Here's how the part is built. I have some questions about the finished solid (model axes, mm). Coordinates: 2 decimals unless noted, no trailing zeros.
from build123d import *

# Parameters (mm, degrees)
F0_W     = 115
F0_H     = 85
F0_W_2   = 3.3230667468
F0_H_2   = 2.7188727399
F0_W_3   = 12.42488157
F0_H_3   = 2.8554350138
F0_W_4   = 2.7188727399
F0_H_4   = 3.3230667468
F0_W_5   = 2.8554350138
F0_H_5   = 12.42488157
F1_DEPTH = 3
F2_R     = 2.6556349186
F3_D     = 3.3
F3_DEPTH = 13.5
F3_TIP   = 0.9914200214
F4_D     = 3.3


with BuildPart() as f1:
    # F0 (on Top) → F1 (new body)
    with BuildSketch(Plane.XY):
        Rectangle(F0_W, F0_H)
        with Locations((-31.5384735586, -39.6359708975)):
            Rectangle(F0_W_2, F0_H_2, mode=Mode.SUBTRACT)
        with Locations((-23.0330330087, -39.6208088496)):
            Rectangle(F0_W_2, F0_H_2, mode=Mode.SUBTRACT)
        with Locations((0.012440607, -39.7679619491)):
            Rectangle(F0_W_3, F0_H_3, mode=Mode.SUBTRACT)
        with Locations((23.7232622458, -35.9257351956)):
            Rectangle(F0_W_2, F0_H_2, mode=Mode.SUBTRACT)
        with Locations((32.2287027957, -35.9105731477)):
            Rectangle(F0_W_2, F0_H_2, mode=Mode.SUBTRACT)
        with Locations((0.0594367157, -4.1384646902)):
            Rectangle(F0_W_4, F0_H_4, mode=Mode.SUBTRACT)
        with Locations((54.6148940921, -0.0461908057)):
            Rectangle(F0_W_5, F0_H_5, mode=Mode.SUBTRACT)
        with Locations((-54.6360462904, 0)):
            Rectangle(F0_W_5, F0_H_5, mode=Mode.SUBTRACT)
        with Locations((-31.1669755029, 39.4913438358)):
            Rectangle(F0_W_2, F0_H_2, mode=Mode.SUBTRACT)
        with Locations((-22.6615349529, 39.5065058838)):
            Rectangle(F0_W_2, F0_H_2, mode=Mode.SUBTRACT)
        with Locations((0.0442746677, 4.3669758597)):
            Rectangle(F0_W_4, F0_H_4, mode=Mode.SUBTRACT)
        with Locations((0.1124413684, 39.7277288139)):
            Rectangle(F0_W_3, F0_H_3, mode=Mode.SUBTRACT)
        with Locations((23.6730267061, 36.7241497734)):
            Rectangle(F0_W_2, F0_H_2, mode=Mode.SUBTRACT)
        with Locations((32.178467256, 36.7393118213)):
            Rectangle(F0_W_2, F0_H_2, mode=Mode.SUBTRACT)
    extrude(amount=-F1_DEPTH)

    # F2
    f2_edges = [f1.edges().sort_by_distance(p)[0] for p in [
        (57.5, -42.5, -1.5),
        (57.5, 42.5, -1.5),
        (-57.5, -42.5, -1.5),
        (-57.5, 42.5, -1.5),
    ]]
    fillet(f2_edges, radius=F2_R)

    # F3
    with Locations(Plane.XY):
        with Locations((-53.4860491753, -38.9412779514), (-53.4860491753, 39.0123836696), (53.5768903792, -38.9412779514), (53.5768903792, 39.0123836696)):
            Hole(F3_D / 2, depth=F3_DEPTH)
            with Locations((0, 0, -(F3_DEPTH + F3_TIP / 2))):  # 118° drill point
                Cone(0, F3_D / 2, F3_TIP, mode=Mode.SUBTRACT)

    # F4 (through all)
    with Locations(Plane.XY):
        with Locations((-41.9517233968, 27.4363141507), (-12.0857078582, 27.4363141507), (-12.0857078582, -27.9048345983), (10.3388316929, 30.7378862053), (45.184802264, 11.4016206935), (45.184802264, -29.8165101558), (10.3388316929, -10.2981757373), (-41.9517233968, -27.9048345983)):
            Hole(F4_D / 2)


solid = f1.part
Q1. We'd pull the mould along X, two halves only. Please class faces 1 (the flat face through (-1, 1, -3)), 2 (the flat face through (0, 2.705, -1)), 3 (the flat face through (-57.5, -1, -1)): pulls with the +X half, pulls with the -X half, needs draft (parallel to the pull), parting line crosses it, or undercut.
Q2. Suppose I cut it at A-A on z = -0.9. State how many separate pieces and enclosed holes the cut face has, and give its area (3 significant figures).
Q3. Please list where these lines run through material, in increasing order: probe 1 along X at (y, z) = (-39, -1.7) (1 decimal); probe 2 along X at (y, z) = (1, -0.7); probe 3 along X at (y, z) = (-37.5, -1.95).
Q4. Will this pin go through, and if not, where does the flat tip stop? P1, Ø3, axis at x = 45.18, y = 11.4, coming from the +Z side.
Check values:
1. face 1: needs draft
1. face 2: undercut
1. face 3: pulls with the -X half
2. separate pieces: 1
2. enclosed holes: 26
2. area: 9,430 mm2
3. probe 1: x = -57.5 to -55.1, -51.8 to -33.2, -29.9 to -24.7, -21.4 to -6.2, 6.2 to 51.9, 55.2 to 57.5
3. probe 2: x = -57.5 to -56.06, -53.21 to 53.19, 56.04 to 57.5
3. probe 3: x = -57.5 to -54.29, -52.68 to 52.77, 54.38 to 57.5
4. P1: passes through
